CAD build for the part. Positions are in the model's coordinates, mm. Give positions to 0.01 mm unless a question says otherwise; leave off trailing zeros. Write each loop counter-clockwise with the first axis right and the second up, starting at its lowest first coordinate (ties: lowest second). Pieces come first, ordered by that corner, then holes. Notation, with made-up numbers: (61, 9.25) - (100, 9.25) arc R17 ccw to (100, 15.25) - close; hole circle Ø6 at (11, 45.5). An arc over 180 degrees is marked (long way). Put each result on its own line as item: value. Start each with the question number.
1. Cut at C-C on x = -1.5. List the corners of the cut face in (y, z) (3 decimals), and give its area (3 significant figures).
2. Cut at B-B on z = 6.35. List the corners of the cut face in (x, y) (3 decimals).
3. Mould opens along X. For faces 1 (the cylindrical face through (0.308, -0.428, 0.798)), 2 (the flat face through (2.781, -1, 5)), 3 (the flat face through (-2, -1, 1.575)), 4 (the flat face through (4.356, 0, 5)) say: +X half, -X half, draft (parallel to the pull), parting line (faces both ways), or undercut.
4. Cut at A-A on y = 0. List the corners of the cut face in (x, z) (1 decimal).
5. Cut at D-D on x = 3.25. List the corners of the cut face in (y, z) (3 decimals), and give its area (3 significant figures).
6. Drop flat-ended pins along their axis: pin 1 (5 mm diameter, centred on x = -0.5, z = 5.5, fed in from +Y); pin 2 (2.5 mm diameter, centred on y = 0, z = 6.35, fed in from -X); pin 3 (3 mm diameter, centred on x = 0.5, y = 0.5, fed in from +Z). Give the stop position or say it passes through.
7. Wall check: line 1 (Y direction, x = 3.55, z = 6.35) (3 decimals); line 2 (X direction, y = 0.25, z = 5); line 3 (Z direction, x = -3.5, y = -2). Give the ranges that are in metal, low to high.
from build123d import *

# Parameters (mm, degrees)
SKETCH1_W           = 8.7122
SKETCH1_H           = 6.35
BOSS_EXTRUDE1_DEPTH = 1.5748
SKETCH2_W           = 1.5748
SKETCH2_H           = 6.35
BOSS_EXTRUDE2_DEPTH = 7.9502
SKETCH3_R           = 1.1176
CUT_EXTRUDE1_DEPTH  = 2.5748
SKETCH4_R           = 1.1176
CUT_EXTRUDE2_DEPTH  = 9.7122


with BuildPart() as part:
    # Sketch1 → Boss-Extrude1 (new body)
    with BuildSketch(Plane.XY):
        Rectangle(SKETCH1_W, SKETCH1_H)
    extrude(amount=BOSS_EXTRUDE1_DEPTH)

    # Sketch2 → Boss-Extrude2 (add)
    with BuildSketch(Plane.XY.offset(1.5748)):
        with Locations((3.5687, 0)):
            Rectangle(SKETCH2_W, SKETCH2_H)
    extrude(amount=BOSS_EXTRUDE2_DEPTH)

    # Sketch3 → Cut-Extrude1 (cut, through all)
    with BuildSketch(Plane.XY.offset(1.5748)):
        with Locations((-0.7239, 0)):
            Circle(SKETCH3_R)
    extrude(amount=-CUT_EXTRUDE1_DEPTH, mode=Mode.SUBTRACT)

    # Sketch4 → Cut-Extrude2 (cut, through all)
    with BuildSketch(Plane(origin=(4.3561, 0, 0), x_dir=(0, 0, -1), z_dir=(1, 0, 0))):
        with Locations((-6.35, 0)):
            Circle(SKETCH4_R)
    extrude(amount=-CUT_EXTRUDE2_DEPTH, mode=Mode.SUBTRACT)


solid = part.part
Report:
1. outline: (-3.175, 0) - (-0.804, 0) - (-0.804, 1.575) - (-3.175, 1.575) - close; (0.804, 0) - (3.175, 0) - (3.175, 1.575) - (0.804, 1.575) - close
1. area: 7.47 mm²
2. outline: (2.781, -3.175) - (4.356, -3.175) - (4.356, -1.118) - (2.781, -1.118) - close; (2.781, 1.118) - (4.356, 1.118) - (4.356, 3.175) - (2.781, 3.175) - close
3. face 1: undercut
3. face 2: -X half
3. face 3: draft
3. face 4: +X half
4. outline: (-4.4, 0) - (-1.8, 0) - (-1.8, 1.6) - (-4.4, 1.6) - close; (0.4, 0) - (4.4, 0) - (4.4, 5.2) - (2.8, 5.2) - (2.8, 1.6) - (0.4, 1.6) - close; (2.8, 7.5) - (4.4, 7.5) - (4.4, 9.5) - (2.8, 9.5) - close
5. outline: (-3.175, 0) - (3.175, 0) - (3.175, 9.525) - (-3.175, 9.525) - close; hole circle Ø2.235 at (0, 6.35)
5. area: 56.6 mm²
6. pin 1: passes through
6. pin 2: stops at x = 2.78
6. pin 3: stops at z = 1.57
7. line 1: y = -3.175 to -1.118, 1.118 to 3.175
7. line 2: x = 2.78 to 4.36
7. line 3: z = 0 to 1.57
